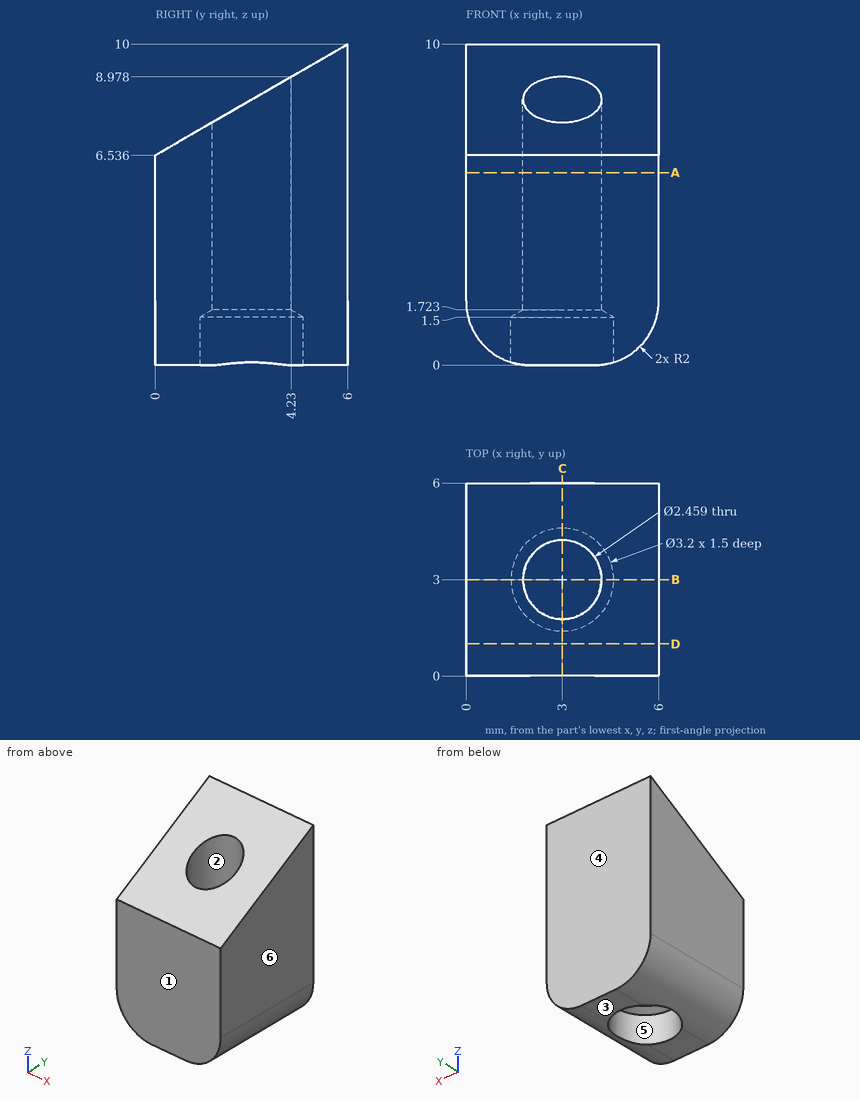
Job drawing, mm, ordinate dimensions from the low corner. One solid piece. A direction names the side the tool comes from. Round coordinates to 2 decimals unless told otherwise and drop trailing zeros. Loops run counter-clockwise (first coordinate to the right, second up) from the corner with the lowest first, then second, coordinate; pieces in that order, holes last.
(1) Cut at D-D (y = 1). Give the cut face in (x, z).
(2) Cut at A-A (z = 6). Give the cut face in (x, y).
(3) Cut at B-B (y = 3). Give the cut face in (x, z).
(4) Wall check: line 1 along X through (y, z) = (3, 5.5); line 2 along X through (y, z) = (3, 0.45) (1 decimal); line 3 along Y through (x, z) = (4, 6.25) (1 decimal). Give the ranges that are in metal, low to high.
(5) Which spindle directions (+Z, -Z, +X, -X, +Y, -Y) get a long thin tool onto all of the face, cutting with end or side? Do the marked faces 5 and 6. Say none if no direction does.
(6) Two-plate mould, pull along Y, no slides. Class the marked faces 1, 2, 3 and 4: +Y half, -Y half, draft (parallel to the pull), parting line (faces both ways), or undercut.
(7) Cut at C-C (x = 3). Give the cut face in (y, z) (1 decimal).
(8) Drop a flat-ended pin along its axis: pin 1 (2 mm diameter, centred on x = 3, y = 3, fed in from +Z). Give the stop position or say it passes through.
Findings below:
1. outline: (0, 2) arc R2 ccw to (2, 0) - (4, 0) arc R2 ccw to (6, 2) - (6, 7.11) - (0, 7.11) - close
2. outline: (0, 0) - (6, 0) - (6, 6) - (0, 6) - close; hole circle Ø2.46 at (3, 3)
3. outline: (0, 2) arc R2 ccw to (1.4, 0.09) - (1.4, 1.5) - (1.77, 1.72) - (1.77, 8.27) - (0, 8.27) - close; (4.23, 1.72) - (4.6, 1.5) - (4.6, 0.09) arc R2 ccw to (6, 2) - (6, 8.27) - (4.23, 8.27) - close
4. line 1: x = 0 to 1.77, 4.23 to 6
4. line 2: x = 0.7 to 1.4, 4.6 to 5.3
4. line 3: y = 0 to 2.3, 3.7 to 6
5. face 5: -Z
5. face 6: +Z, -Z, +X, +Y, -Y
6. face 1: -Y half
6. face 2: undercut
6. face 3: draft
6. face 4: +Y half
7. outline: (0, 0) - (1.4, 0) - (1.4, 1.5) - (1.8, 1.7) - (1.8, 7.6) - (0, 6.5) - close; (4.2, 1.7) - (4.6, 1.5) - (4.6, 0) - (6, 0) - (6, 10) - (4.2, 9) - close
8. pin 1: passes through
